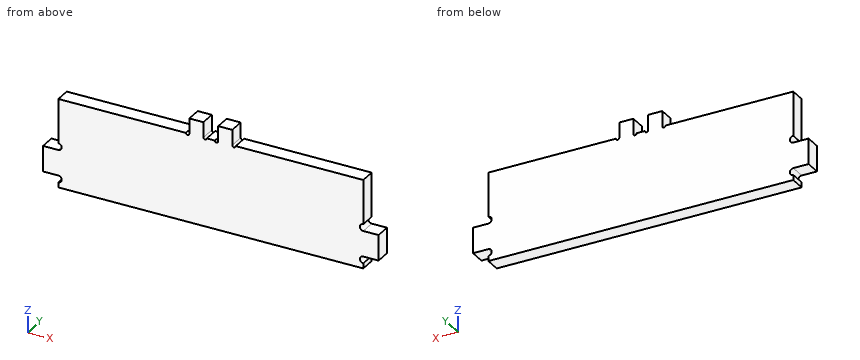
Autodesk Inventor part; units mm, degrees
ref_plane "YZ Plane" through (0, 0, 0) normal (1, 0, 0) x (0, 1, 0)
ref_plane "XZ Plane" through (0, 0, 0) normal (0, 1, 0) x (-1, 0, 0)
ref_plane "XY Plane" through (0, 0, 0) normal (0, 0, 1) x (1, 0, 0)
sketch "Sketch1" plane through (0, 0, 0) normal (0, 1, 0) x (-1, 0, 0)
  line L0 (54.4292, -43.2642) -> (54.4292, -41.2642)
  arc A0 (54.4292, -38.5976) -> (54.4292, -41.2642) centre (54.4292, -39.9309) ccw
  arc A1 (54.4292, -25.9309) -> (54.4292, -28.5976) centre (54.4292, -27.2642) ccw
  line L1 (54.4292, -25.9309) -> (54.4292, -8.5976)
  line L2 (54.4292, -28.5976) -> (60.4292, -28.5976)
  line L3 (54.4292, -38.5976) -> (60.4292, -38.5976)
  line L4 (60.4292, -38.5976) -> (60.4292, -28.5976)
  line L5 (54.4292, -43.2642) -> (-65.0708, -43.2642)
  line L6 (-65.0708, -43.2642) -> (-65.0708, -41.2642)
  arc A2 (-65.0708, -41.2642) -> (-65.0708, -38.5976) centre (-65.0708, -39.9309) ccw
  arc A3 (-65.0708, -28.5976) -> (-65.0708, -25.9309) centre (-65.0708, -27.2642) ccw
  line L7 (-65.0708, -25.9309) -> (-65.0708, -8.5976)
  line L8 (-65.0708, -28.5976) -> (-71.0708, -28.5976)
  line L9 (-65.0708, -38.5976) -> (-71.0708, -38.5976)
  line L10 (-71.0708, -38.5976) -> (-71.0708, -28.5976)
  line L11 (-21.0708, -8.5976) -> (-65.0708, -8.5976)
  line L12 (54.4292, -8.5976) -> (10.4292, -8.5976)
  line L13 (-19.7375, -2.5976) -> (9.0959, -2.5976)
  line L14 (-19.7375, -8.5976) -> (-19.7375, -2.5976)
  line L15 (9.0959, -8.5976) -> (9.0959, -2.5976)
  line L16 (-21.0708, -8.5976) -> (-19.7375, -8.5976)
  line L17 (10.4292, -8.5976) -> (9.0959, -8.5976)
  point P0 (0, 0)
  dimension "d1" = 2
  dimension "d2" = 2.6667
  dimension "d5" = 2.6667
  dimension "d6" = 17.3333
  dimension "d9" = 6
  dimension "d10" = 119.5
  dimension "d11" = 10
  dimension "d18" = 44
  dimension "d19" = 44
  dimension "d21" = 20
  dimension "d23" = 6
extrude "Extrusion1" add sketch "Sketch1" along normal blind 6
sketch "Sketch2" plane through (0, 6, 0) normal (0, 1, 0) x (1, 0, 0)
  line L0 (2.4041, 2.5976) -> (2.4041, 8.5976)
  line L1 (-3.0959, 8.5976) -> (-3.0959, 2.5976)
  line L2 (-9.0959, 8.5976) -> (-9.0959, 2.5976)
  line L3 (13.7375, 8.5976) -> (13.7375, 2.5976)
  line L4 (8.2375, 2.5976) -> (8.2375, 8.5976)
  line L5 (19.7375, 2.5976) -> (19.7375, 8.5976)
  line L6 (-9.0959, 8.5976) -> (-4.4292, 8.5976)
  line L7 (-3.0959, 8.5976) -> (-3.0959, 2.5976)
  line L8 (-3.0959, 2.5976) -> (-9.0959, 2.5976)
  line L9 (-9.0959, 2.5976) -> (-9.0959, 8.5976)
  line L10 (3.7375, 8.5976) -> (6.9041, 8.5976)
  line L11 (8.2375, 8.5976) -> (8.2375, 2.5976)
  line L12 (8.2375, 2.5976) -> (2.4041, 2.5976)
  line L13 (2.4041, 2.5976) -> (2.4041, 8.5976)
  line L14 (15.0708, 8.5976) -> (19.7375, 8.5976)
  line L15 (19.7375, 8.5976) -> (19.7375, 2.5976)
  line L16 (19.7375, 2.5976) -> (13.7375, 2.5976)
  line L17 (13.7375, 2.5976) -> (13.7375, 8.5976)
  arc A0 (3.7375, 8.5976) -> (2.4041, 8.5976) centre (3.0708, 8.5976) ccw
  arc A1 (8.2375, 8.5976) -> (6.9041, 8.5976) centre (7.5708, 8.5976) ccw
  arc A2 (-3.0959, 8.5976) -> (-4.4292, 8.5976) centre (-3.7625, 8.5976) ccw
  arc A3 (15.0708, 8.5976) -> (13.7375, 8.5976) centre (14.4041, 8.5976) ccw
  point P0 (0, 0)
  dimension "d26" = 6
  dimension "d28" = 6
  dimension "d29" = 6
  dimension "d37" = 1.3333
  dimension "d38" = 1.3333
  dimension "d39" = 1.3333
  dimension "d40" = 1.3333
extrude "Extrusion2" cut sketch "Sketch2" against normal through all
properties part number "Support A Cross Dual2" material "Wood (Maple)"
Input: part model. Units: mm. Frame: model coordinates. Give positions to 0.01 mm unless a question says otherwise; leave off trailing zeros. Loops run counter-clockwise (first coordinate to the right, second up) from the corner with the lowest first, then second, coordinate; pieces in that order, holes last. Notation, with made-up numbers: (83.5, 14.25) - (120.5, 14.25) arc R31 ccw to (120.5, 49.25) - close; hole circle Ø11 at (55.5, -18). An arc over 180 degrees is marked (long way). Use CSV: the item, a comma, the result in double quotes. Start each with the question number.
Item 1: Line query: line 1 (Z direction, x = 28.5, y = 5.35); line 2 (X direction, y = 5, z = -23); line 3 (X direction, y = 0.5, z = -27). Output: solid intervals per line, ascending.
Item 2: Section B-B on y = 3.2. Return loops of the section in (x, z).
Item 3: Section C-C on z = -17. Return loops of the section in (x, y), then the cut area to 3 significant figures.
Item 4: Section D-D on x = -27.5. Return loops of the section in (y, z).
Item 5: Section A-A on z = -7. Return loops of the section in (x, y).
Item 6: Contact query for flat-ended pins moving along their axis: P1, Ø2.5, axis at x = 5.5, y = 2.5, coming from the +Z side; P2, Ø1.6, axis at y = 4, z = -42.5, coming from the +X side; P3, Ø1.5, axis at y = 2.5, z = -18.5, coming from the -X side. Output: stop coordinate, or through.
Ans:
1,line 1,"z = -43.26 to -8.6"
1,line 2,"x = -54.43 to 65.07"
1,line 3,"x = -53.12 to 63.76"
2,outline,"(-60.43, -38.6) - (-54.43, -38.6) arc R1.33 cw to (-54.43, -41.26) - (-54.43, -43.26) - (65.07, -43.26) - (65.07, -41.26) arc R1.33 cw to (65.07, -38.6) - (71.07, -38.6) - (71.07, -28.6) - (65.07, -28.6) arc R1.33 cw to (65.07, -25.93) - (65.07, -8.6) - (15.07, -8.6) arc R0.67 cw to (13.74, -8.6) - (13.74, -2.6) - (8.24, -2.6) - (8.24, -8.6) arc R0.67 cw to (6.9, -8.6) - (3.74, -8.6) arc R0.67 cw to (2.4, -8.6) - (2.4, -2.6) - (-3.1, -2.6) - (-3.1, -8.6) arc R0.67 cw to (-4.43, -8.6) - (-54.43, -8.6) - (-54.43, -25.93) arc R1.33 cw to (-54.43, -28.6) - (-60.43, -28.6) - close"
3,outline,"(-54.43, 0) - (65.07, 0) - (65.07, 6) - (-54.43, 6) - close"
3,area,"717 mm2"
4,outline,"(0, -43.26) - (6, -43.26) - (6, -8.6) - (0, -8.6) - close"
5,outline,"(-3.1, 0) - (2.4, 0) - (2.4, 6) - (-3.1, 6) - close; (8.24, 0) - (13.74, 0) - (13.74, 6) - (8.24, 6) - close"
6,P1,"stops at z = -8.6"
6,P2,"stops at x = 65.07"
6,P3,"stops at x = -54.43"
